Geometry: final body of the model. Coordinates: model frame, mm. Round coordinates to 2 decimals unless told otherwise and drop trailing zeros. Loops run counter-clockwise (first coordinate to the right, second up) from the corner with the lowest first, then second, coordinate; pieces in that order, holes last. Notation, with made-up numbers: M 43,60.25 L 86,60.25 A15 ccw 86,84.25 Z; hole C 46,87 d5. An arc over 180 degrees is marked long. Return JSON: item names as keys, results as strings.
from build123d import *

# Parameters (mm, degrees)
F0_R     = 1.6256
F1_DEPTH = 25.4
F2_R     = 5.08
F3_R     = 3.81


with BuildPart() as f1:
    # F0 (on Front) → F1 (new body)
    with BuildSketch(Plane.XZ):
        with BuildLine():
            Line((-10.059392821, 9.5458903177), (-10.059392821, 3.5927653177))
            ThreePointArc((-10.059392821, 3.5927653177), (-8.3157628778, 7.8022603745), (-4.106267821, 9.5458903177))
            Line((-4.106267821, 9.5458903177), (-10.059392821, 9.5458903177))
        make_face()
        with BuildLine():
            ThreePointArc((-4.106267821, 9.5458903177), (-8.3157628778, 7.8022603745), (-10.059392821, 3.5927653177))
            ThreePointArc((-10.059392821, 3.5927653177), (-8.3157628778, -0.616729739), (-4.106267821, -2.3603596823))
            ThreePointArc((-4.106267821, -2.3603596823), (0.1032272357, -0.616729739), (1.846857179, 3.5927653177))
            ThreePointArc((1.846857179, 3.5927653177), (0.1032272357, 7.8022603745), (-4.106267821, 9.5458903177))
        make_face()
        with Locations((-4.106267821, 3.5927653177)):
            Circle(F0_R, mode=Mode.SUBTRACT)
        with BuildLine():
            Line((1.846857179, 9.5458903177), (-4.106267821, 9.5458903177))
            ThreePointArc((-4.106267821, 9.5458903177), (0.1032272357, 7.8022603745), (1.846857179, 3.5927653177))
            Line((1.846857179, 3.5927653177), (1.846857179, 9.5458903177))
        make_face()
        with BuildLine():
            ThreePointArc((1.846857179, 3.5927653177), (0.1032272357, -0.616729739), (-4.106267821, -2.3603596823))
            Line((-4.106267821, -2.3603596823), (1.846857179, -2.3603596823))
            Line((1.846857179, -2.3603596823), (1.846857179, 3.5927653177))
        make_face()
        with BuildLine():
            ThreePointArc((-4.106267821, -2.3603596823), (-8.3157628778, -0.616729739), (-10.059392821, 3.5927653177))
            Line((-10.059392821, 3.5927653177), (-10.059392821, -2.3603596823))
            Line((-10.059392821, -2.3603596823), (-4.106267821, -2.3603596823))
        make_face()
    extrude(amount=F1_DEPTH)

    # F2
    f2_edges = [f1.edges().sort_by_distance(p)[0] for p in [
        (1.846857, -12.7, 9.54589),
        (-10.059393, -12.7, 9.54589),
    ]]
    fillet(f2_edges, radius=F2_R)

    # F3
    f3_edges = [f1.edges().sort_by_distance(p)[0] for p in [
        (-10.059393, -12.7, -2.36036),
        (1.846857, -12.7, -2.36036),
    ]]
    fillet(f3_edges, radius=F3_R)


solid = f1.part
Q1. Section query B-B (y = -9.5). Output: boundary loops of the cut face in (x, z), plus the area to 3 significant figures.
Determined:
{"outline": "M -10.06,1.45 A3.81 ccw -6.25,-2.36 L -1.96,-2.36 A3.81 ccw 1.85,1.45 L 1.85,4.47 A5.08 ccw -3.23,9.55 L -4.98,9.55 A5.08 ccw -10.06,4.47 Z; hole C -4.11,3.59 d3.25", "area": "116 mm^2"}
Q2. Section query A-A (x = -3.5). Output: boundary loops of the cut face in (y, z), plus the area to 3 significant figures.
Determined:
{"outline": "M -25.4,-2.36 L 0,-2.36 L 0,2.08 L -25.4,2.08 Z; M -25.4,5.1 L 0,5.1 L 0,9.55 L -25.4,9.55 Z", "area": "226 mm^2"}
Q3. Section query D-D (z = 7.5). Output: boundary loops of the cut face in (x, y), plus the area to 3 significant figures.
Determined:
{"outline": "M -9.05,-25.4 L 0.84,-25.4 L 0.84,0 L -9.05,0 Z", "area": "251 mm^2"}
Q4. Section query C-C (z = 4). Output: boundary loops of the cut face in (x, y), plus the area to 3 significant figures.
Determined:
{"outline": "M -10.06,-25.4 L -5.68,-25.4 L -5.68,0 L -10.06,0 Z; M -2.53,-25.4 L 1.85,-25.4 L 1.85,0 L -2.53,0 Z", "area": "222 mm^2"}
Q5. Pull-direction query (Z, two-part tool) for faces 1 (the flat face through (-4, -13, -2.36)), 2 (the flat face through (-3, -25.4, 2)), 3 (the cylindrical face through (-4.459, -12.522, 2.006)), 4 (the cylindrical face through (0.398, -12.878, 8.018)); classes: pulls with the +Z half, pulls with the -Z half, needs draft (parallel to the pull), parting line crosses it, or undercut.
Determined:
{"face 1": "pulls with the -Z half", "face 2": "needs draft", "face 3": "undercut", "face 4": "pulls with the +Z half"}
Q6. Material intervals for L1, parallel to Z at x = -4, y = -8.75; L2, parallel to X at y = -5, z = 1.25; L3, parallel to X at y = -19.5, z = 2.75, sorted ascending.
Determined:
{"L1": "z = -2.36 to 1.97, 5.21 to 9.55", "L2": "x = -10.05 to 1.84", "L3": "x = -10.06 to -5.5, -2.72 to 1.85"}
